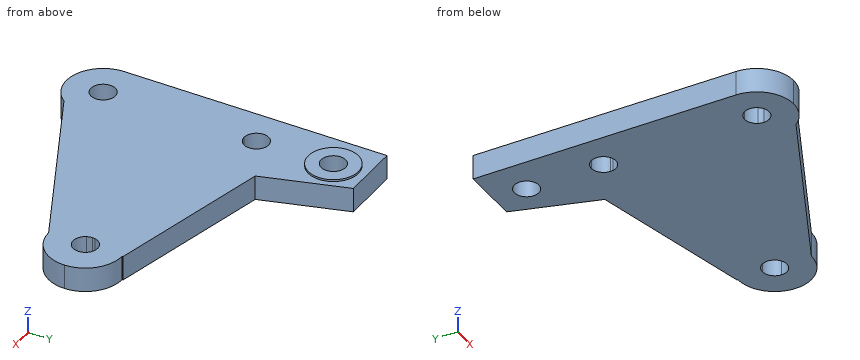
from build123d import *

# Parameters (mm, degrees)
F1_DEPTH = 6.35
F2_R     = 3.175
F3_DEPTH = 12.7
F4_R     = 6.4822420389
F5_DEPTH = 6.35
F6_DEPTH = 19.558
F7_DEPTH = 6.35
F8_R     = 6.4822420389
F8_R_2   = 3.175
F9_DEPTH = 6.35


with BuildPart() as f1:
    # F0 (on Top) → F1 (new body)
    with BuildSketch(Plane.XY):
        with BuildLine():
            Line((0, -17.430102046), (0, 0))
            Line((0, 0), (0, 3.216402))
            ThreePointArc((0, 3.216402), (-6.7351920908, 6.0062099092), (-9.525, 12.741402))
            Line((-9.525, 12.741402), (-9.525, -26.955102046))
            ThreePointArc((-9.525, -26.955102046), (-6.7351920908, -20.2199099552), (0, -17.430102046))
        make_face()
        with BuildLine():
            ThreePointArc((-9.525, 12.741402), (-6.7351920908, 6.0062099092), (0, 3.216402))
            Line((0, 3.216402), (0, 9.566402))
            ThreePointArc((0, 9.566402), (-3.175, 12.741402), (0, 15.916402))
            Line((0, 15.916402), (0, 22.266402))
            ThreePointArc((0, 22.266402), (-6.7351920908, 19.4765940908), (-9.525, 12.741402))
        make_face()
        with BuildLine():
            Line((0, -23.780102046), (0, -17.430102046))
            ThreePointArc((0, -17.430102046), (-6.7351920908, -20.2199099552), (-9.525, -26.955102046))
            ThreePointArc((-9.525, -26.955102046), (-6.7351920908, -33.6902941368), (0, -36.480102046))
            Line((0, -36.480102046), (7.5123847033, -32.8108429103))
            ThreePointArc((7.5123847033, -32.8108429103), (9.007804652, -30.0510801387), (9.525, -26.955102046))
            ThreePointArc((9.525, -26.955102046), (9.2802728088, -24.809837122), (8.5586668568, -22.7748093967))
            Line((8.5586668568, -22.7748093967), (2.8528889523, -25.5616711629))
            ThreePointArc((2.8528889523, -25.5616711629), (3.0934242696, -26.240013738), (3.175, -26.955102046))
            ThreePointArc((3.175, -26.955102046), (-2.2450640303, -29.2001660763), (0, -23.780102046))
        make_face()
        with BuildLine():
            ThreePointArc((9.525, 12.741402), (9.463768469, 11.6631110537), (9.2808611307, 10.5986837096))
            Line((9.2808611307, 10.5986837096), (45.9066000969, 2.1427182904))
            ThreePointArc((45.9066000969, 2.1427182904), (49.2580332078, 7.4543617002), (55.1874612276, 9.525))
            Line((55.1874612276, 9.525), (55.1874612276, 9.7662775009))
            Line((55.1874612276, 9.7662775009), (4.1043156247, 21.3367622748))
            ThreePointArc((4.1043156247, 21.3367622748), (8.0566503997, 17.8223477129), (9.525, 12.741402))
        make_face()
        with BuildLine():
            Line((3.0936203769, 12.0271625699), (9.2808611307, 10.5986837096))
            ThreePointArc((9.2808611307, 10.5986837096), (9.463768469, 11.6631110537), (9.525, 12.741402))
            ThreePointArc((9.525, 12.741402), (8.0566503997, 17.8223477129), (4.1043156247, 21.3367622748))
            Line((4.1043156247, 21.3367622748), (0, 22.266402))
            Line((0, 22.266402), (0, 15.916402))
            ThreePointArc((0, 15.916402), (2.2450640303, 14.9864660303), (3.175, 12.741402))
            ThreePointArc((3.175, 12.741402), (3.1545894897, 12.3819716846), (3.0936203769, 12.0271625699))
        make_face()
        with BuildLine():
            ThreePointArc((55.1874612276, 9.525), (49.2580332078, 7.4543617002), (45.9066000969, 2.1427182904))
            Line((45.9066000969, 2.1427182904), (52.0938408507, 0.7142394301))
            ThreePointArc((52.0938408507, 0.7142394301), (53.210985221, 2.4847872334), (55.1874612276, 3.175))
            Line((55.1874612276, 3.175), (55.1874612276, 9.525))
        make_face()
        with BuildLine():
            ThreePointArc((55.1874612276, -9.525), (50.1422487685, -8.0790752096), (46.6287943708, -4.1802926493))
            Line((46.6287943708, -4.1802926493), (8.5586668568, -22.7748093967))
            ThreePointArc((8.5586668568, -22.7748093967), (9.2802728088, -24.809837122), (9.525, -26.955102046))
            ThreePointArc((9.525, -26.955102046), (9.007804652, -30.0510801387), (7.5123847033, -32.8108429103))
            Line((7.5123847033, -32.8108429103), (55.1874612276, -9.525))
        make_face()
        with BuildLine():
            Line((52.3345722753, -1.3934308831), (46.6287943708, -4.1802926493))
            ThreePointArc((46.6287943708, -4.1802926493), (50.1422487685, -8.0790752096), (55.1874612276, -9.525))
            ThreePointArc((55.1874612276, -9.525), (61.9226533184, -6.7351920908), (64.7124612276, 0))
            ThreePointArc((64.7124612276, 0), (61.9226533184, 6.7351920908), (55.1874612276, 9.525))
            Line((55.1874612276, 9.525), (55.1874612276, 3.175))
            ThreePointArc((55.1874612276, 3.175), (57.4325252579, 2.2450640303), (58.3624612276, 0))
            ThreePointArc((58.3624612276, 0), (55.9025495356, -3.0934242696), (52.3345722753, -1.3934308831))
        make_face()
        with BuildLine():
            ThreePointArc((4.1043156247, 21.3367622748), (2.1041409628, 22.0310852997), (0, 22.266402))
            Line((0, 22.266402), (4.1043156247, 21.3367622748))
        make_face()
        with BuildLine():
            Line((7.5123847033, -32.8108429103), (0, -36.480102046))
            ThreePointArc((0, -36.480102046), (4.1802926493, -35.5137689028), (7.5123847033, -32.8108429103))
        make_face()
        with BuildLine():
            Line((0, 3.216402), (0, 0))
            Line((0, 0), (45.6624612276, 0))
            ThreePointArc((45.6624612276, 0), (45.7236927586, 1.0782909463), (45.9066000969, 2.1427182904))
            Line((45.9066000969, 2.1427182904), (9.2808611307, 10.5986837096))
            ThreePointArc((9.2808611307, 10.5986837096), (5.9294280198, 5.2870402998), (0, 3.216402))
        make_face()
        with BuildLine():
            Line((0, 9.566402), (0, 3.216402))
            ThreePointArc((0, 3.216402), (5.9294280198, 5.2870402998), (9.2808611307, 10.5986837096))
            Line((9.2808611307, 10.5986837096), (3.0936203769, 12.0271625699))
            ThreePointArc((3.0936203769, 12.0271625699), (1.9764760066, 10.2566147666), (0, 9.566402))
        make_face()
        with BuildLine():
            Line((45.6624612276, 0), (0, 0))
            Line((0, 0), (0, -17.430102046))
            ThreePointArc((0, -17.430102046), (5.0452124591, -18.8760268364), (8.5586668568, -22.7748093967))
            Line((8.5586668568, -22.7748093967), (46.6287943708, -4.1802926493))
            ThreePointArc((46.6287943708, -4.1802926493), (45.9071884188, -2.145264924), (45.6624612276, 0))
        make_face()
        with BuildLine():
            ThreePointArc((8.5586668568, -22.7748093967), (5.0452124591, -18.8760268364), (0, -17.430102046))
            Line((0, -17.430102046), (0, -23.780102046))
            ThreePointArc((0, -23.780102046), (1.6817374864, -24.2620769761), (2.8528889523, -25.5616711629))
            Line((2.8528889523, -25.5616711629), (8.5586668568, -22.7748093967))
        make_face()
        with BuildLine():
            Line((52.0124612276, 0), (45.6624612276, 0))
            ThreePointArc((45.6624612276, 0), (45.9071884188, -2.145264924), (46.6287943708, -4.1802926493))
            Line((46.6287943708, -4.1802926493), (52.3345722753, -1.3934308831))
            ThreePointArc((52.3345722753, -1.3934308831), (52.094036958, -0.715088308), (52.0124612276, 0))
        make_face()
        with BuildLine():
            ThreePointArc((45.9066000969, 2.1427182904), (45.7236927586, 1.0782909463), (45.6624612276, 0))
            Line((45.6624612276, 0), (52.0124612276, 0))
            ThreePointArc((52.0124612276, 0), (52.0328717379, 0.3594303154), (52.0938408507, 0.7142394301))
            Line((52.0938408507, 0.7142394301), (45.9066000969, 2.1427182904))
        make_face()
    extrude(amount=F1_DEPTH)

    # F2 (on face) → F3 (join)
    with BuildSketch(Plane.XY.offset(6.35)):
        with BuildLine():
            Line((-9.525, 41.1111302674), (-9.525, 12.741402))
            ThreePointArc((-9.525, 12.741402), (-5.0809457129, 20.7980523997), (4.1043156247, 21.3367622748))
            Line((4.1043156247, 21.3367622748), (12.3195811982, 19.4759801301))
            Line((12.3195811982, 19.4759801301), (5.7150009088, 41.1111302674))
            Line((5.7150009088, 41.1111302674), (-9.525, 41.1111302674))
        make_face()
        with Locations((-0.0769013266, 32.6290909023)):
            Circle(F2_R, mode=Mode.SUBTRACT)
    extrude(amount=-F3_DEPTH)

    # F4 (on face) → F5 (cut)
    with BuildSketch(Plane(origin=(0, 0, -6.35), x_dir=(1, 0, 0), z_dir=(0, 0, -1))):
        with BuildLine():
            Line((-9.525, -41.1111302674), (5.7150009088, -41.1111302674))
            Line((5.7150009088, -41.1111302674), (12.3195811982, -19.4759801301))
            Line((12.3195811982, -19.4759801301), (4.1043156247, -21.3367622748))
            ThreePointArc((4.1043156247, -21.3367622748), (-5.0809457129, -20.7980523997), (-9.525, -12.741402))
            Line((-9.525, -12.741402), (-9.525, -41.1111302674))
        make_face()
        with Locations((-0.0769013266, -32.6290909023)):
            Circle(F4_R, mode=Mode.SUBTRACT)
    extrude(amount=-F5_DEPTH, mode=Mode.SUBTRACT)

    # F6 (add): a face of the model
    f6_faces = [f1.faces().sort_by_distance(p)[0] for p in [
        (-6.3757978733, 32.6290909023, -6.35),
    ]]
    extrude(f6_faces, amount=-F6_DEPTH)

    # F7 (cut): a face of the model
    f7_faces = [f1.faces().sort_by_distance(p)[0] for p in [
        (-6.3757978733, 32.6290909023, -6.35),
    ]]
    extrude(f7_faces, amount=-F7_DEPTH, mode=Mode.SUBTRACT)

    # F8 (on face) → F9 (cut)
    with BuildSketch(Plane.XY.offset(13.208)):
        with Locations((-0.0769013266, 32.6290909023)):
            Circle(F8_R)
        with Locations((-0.0769013266, 32.6290909023)):
            Circle(F8_R_2, mode=Mode.SUBTRACT)
    extrude(amount=-F9_DEPTH, mode=Mode.SUBTRACT)


solid = f1.part
Design review of the part built by this model. Coordinates are the model's own, in mm. Round coordinates to 2 decimals unless told otherwise and drop trailing zeros. Write each loop counter-clockwise with the first axis right and the second up, starting at its lowest first coordinate (ties: lowest second). Pieces come first, ordered by that corner, then holes. Notation, with made-up numbers: (10, 45) -> (41, 45) arc R18 cw to (41, 65) -> close; hole circle Ø3 at (59, 44). An arc over 180 degrees is marked (long way). One line per question, with ' | ' between items.
(1) Insertion check: P1, Ø1, axis at x = 55, z = 2, coming from the +Y side; P2, Ø22.5, axis at x = 13.5, y = -11.5, coming from the +Z side; P3, Ø6, axis at x = 3.5, y = -17.5, coming from the -Z side; P4, Ø2, axis at y = 5, z = 6, coming from the +X side. Each pin has a flat end and moves straight along its axis. Give the tip position at first contact, or say it passes through.
Result sheet:
P1: y = 9.92 | P2: z = 6.35 | P3: z = 0 | P4: x = 63.83
(2) Take a section at A-A, the plane x = 53.5. State the section outline as (y, z) points.
Result sheet:
outline: (-10.35, 0) -> (-2.69, 0) -> (-2.69, 6.35) -> (-10.35, 6.35) -> close; (2.69, 0) -> (10.15, 0) -> (10.15, 6.35) -> (2.69, 6.35) -> close
(3) Take a section at C-C, the plane x = 21.5. State the section outline as (y, z) points.
Result sheet:
outline: (-25.98, 0) -> (17.4, 0) -> (17.4, 6.35) -> (-25.98, 6.35) -> close
(4) Wall thickness on line 1 (Z direction, x = 24, y = -4); line 2 (Y direction, x = -2.5, z = 1); line 3 (X direction, y = 30, z = 4) (3 decimals): over which ranges is each line inside the solid? List them lowest first. Write a range as [from, to].
Result sheet:
line 1: [0, 6.35] | line 2: [-36.15, -28.91], [-25, 10.78], [14.7, 30.58], [34.68, 41.11] | line 3: [-9.525, -1.857], [1.703, 9.107]
(5) Take a section at B-B, the plane y = 5. State the section outline as (x, z) points (3 decimals).
Result sheet:
outline: (-9.525, 0) -> (63.295, 0) -> (63.295, 6.35) -> (-9.525, 6.35) -> close
